from build123d import *

# Parameters (mm, degrees)
SKETCH1_W           = 133
SKETCH1_H           = 110
BOSS_EXTRUDE1_DEPTH = 3
SKETCH2_W           = 50
SKETCH2_H           = 18
SKETCH2_W_2         = 41
SKETCH2_H_2         = 15
SKETCH2_W_3         = 31
BOSS_EXTRUDE2_DEPTH = 3
CUT_EXTRUDE1_REACH  = 8
SKETCH3_R           = 15.25
SKETCH4_R           = 16.375
CUT_EXTRUDE2_DEPTH  = 1
CUT_EXTRUDE3_DEPTH  = 7
SKETCH7_W           = 15.45
SKETCH7_H           = 16.15
CUT_EXTRUDE4_DEPTH  = 1.5


with BuildPart() as part:
    # Sketch1 → Boss-Extrude1 (new body)
    with BuildSketch(Plane(origin=(0, 0, 0), x_dir=(1, 0, 0), z_dir=(0, 1, 0))):
        with Locations((66.5, 55)):
            Rectangle(SKETCH1_W, SKETCH1_H)
    extrude(amount=BOSS_EXTRUDE1_DEPTH)

    # Sketch2 → Boss-Extrude2 (add)
    with BuildSketch(Plane.XZ):
        with Locations((25, -109)):
            Rectangle(SKETCH2_W, SKETCH2_H)
        with Locations((112.5, -2.5)):
            Rectangle(SKETCH2_W_2, SKETCH2_H_2)
        with Locations((23.5, -2.5)):
            Rectangle(SKETCH2_W_3, SKETCH2_H_2)
    extrude(amount=BOSS_EXTRUDE2_DEPTH)

    # Sketch3 → Cut-Extrude1 (cut, up to next)
    with BuildSketch(Plane(origin=(0, 3, 0), x_dir=(1, 0, 0), z_dir=(0, 1, 0)), mode=Mode.PRIVATE) as cut_extrude1_sk1:
        with Locations((128.5, 28.75)):
            Circle(SKETCH3_R)
    cut_extrude1_tool1 = extrude(cut_extrude1_sk1.sketch, amount=-CUT_EXTRUDE1_REACH, mode=Mode.PRIVATE) & part.part
    add(cut_extrude1_tool1.solids().sort_by_distance((128.5, 3, -28.75))[0], mode=Mode.SUBTRACT)
    # Sketch3 → Cut-Extrude1 (cut, up to next)
    with BuildSketch(Plane(origin=(0, 3, 0), x_dir=(1, 0, 0), z_dir=(0, 1, 0)), mode=Mode.PRIVATE) as cut_extrude1_sk2:
        with Locations((135.5, 67.25)):
            Circle(SKETCH3_R)
    cut_extrude1_tool2 = extrude(cut_extrude1_sk2.sketch, amount=-CUT_EXTRUDE1_REACH, mode=Mode.PRIVATE) & part.part
    add(cut_extrude1_tool2.solids().sort_by_distance((135.5, 3, -67.25))[0], mode=Mode.SUBTRACT)

    # Sketch4 → Cut-Extrude2 (cut)
    with BuildSketch(Plane.XZ):
        with Locations((128.5, -28.75)):
            Circle(SKETCH4_R)
        with Locations((135.5, -67.25)):
            Circle(SKETCH4_R)
    extrude(amount=-CUT_EXTRUDE2_DEPTH, mode=Mode.SUBTRACT)

    # Sketch6 → Cut-Extrude3 (cut, through all)
    with BuildSketch(Plane(origin=(0, 3, 0), x_dir=(1, 0, 0), z_dir=(0, 1, 0))):
        Polygon((29.575, 84.225), (29.575, 78.275), (28.775, 78.275), (28.775, 74.175), (44.225, 74.175), (44.225, 78.275), (43.425, 78.275), (43.425, 84.225), (44.225, 84.225), (44.225, 88.325), (28.775, 88.325), (28.775, 84.225), align=None)
        Polygon((49.575, 84.225), (49.575, 78.275), (48.775, 78.275), (48.775, 74.175), (64.225, 74.175), (64.225, 78.275), (63.425, 78.275), (63.425, 84.225), (64.225, 84.225), (64.225, 88.325), (48.775, 88.325), (48.775, 84.225), align=None)
        Polygon((69.575, 79.225), (69.575, 73.275), (68.775, 73.275), (68.775, 69.175), (84.225, 69.175), (84.225, 73.275), (83.425, 73.275), (83.425, 79.225), (84.225, 79.225), (84.225, 83.325), (68.775, 83.325), (68.775, 79.225), align=None)
        Polygon((89.575, 39.225), (89.575, 33.275), (88.775, 33.275), (88.775, 29.175), (104.225, 29.175), (104.225, 33.275), (103.425, 33.275), (103.425, 39.225), (104.225, 39.225), (104.225, 43.325), (88.775, 43.325), (88.775, 39.225), align=None)
    extrude(amount=-CUT_EXTRUDE3_DEPTH, mode=Mode.SUBTRACT)

    # Sketch7 → Cut-Extrude4 (cut)
    with BuildSketch(Plane.XZ):
        with Locations((76.5, -76.25)):
            Rectangle(SKETCH7_W, SKETCH7_H)
        with Locations((96.5, -36.25)):
            Rectangle(SKETCH7_W, SKETCH7_H)
        with Locations((56.5, -81.25)):
            Rectangle(SKETCH7_W, SKETCH7_H)
        with Locations((36.5, -81.25)):
            Rectangle(SKETCH7_W, SKETCH7_H)
    extrude(amount=-CUT_EXTRUDE4_DEPTH, mode=Mode.SUBTRACT)


solid = part.part
The listing builds one solid part. Answer for the finished solid, in the listing's coordinates (mm). A direction names the side the tool comes from. Give positions to 0.01 mm unless a question says otherwise; leave off trailing zeros. Write each loop counter-clockwise with the first axis right and the second up, starting at its lowest first coordinate (ties: lowest second). Pieces come first, ordered by that corner, then holes. Notation, with made-up numbers: (47.25, 26) - (97.25, 26) arc R27 cw to (97.25, 45) - close; hole circle Ø11 at (-9.5, -5). An arc over 180 degrees is marked (long way). One line per question, with ' | ' between items. Start each with the question number.
1. Determine the mould class of faces 6 (the face through (112, -1, -10)), 7 (the face through (8, -1, -3)), 8 (the face through (120.253, 2.014, -67.55)), 9 (the face through (39, -1, -3)) for opening direction X: +X half, -X half, draft (parallel to the pull), parting line (faces both ways), or undercut.
2. For faces 1 (the face through (119.13, 0.49, -66.93)), 2 (the face through (25, 0, -114)), 3 (the face through (104.225, 1, -36)), 4 (the face through (25, -1, -100)), 5 (the face through (66, 1, 0)), determine the directions among +Z, -Z, +X, -X, +Y, -Y from which every point of the face is accessible in a straight line to the end or side of a thin tool.
3. Straight lines are drawn through the part: line 1 (Z direction, x = 10.5, y = -1.2); line 2 (Z direction, x = 94, y = 0.95) (3 decimals); line 3 (Z direction, x = 128.5, y = 0.7) (3 decimals). For each, find the intervals that lie inside material, in ascending order.
4. Section D-D, the plane z = -92 is taken. Determine the outline of the cut face in (x, y), then the cut area to 3 significant figures.
5. Section C-C, the plane z = -31.5 is taken. Determine the outline of the cut face in (x, y) (3 decimals), then the cut area to 3 significant figures.
6. Given P1, Ø1.2, axis at x = 37.5, y = 2.5, coming from the +Z side; P2, Ø1.5, axis at y = 2, z = -76.5, coming from the +X side; P3, Ø6, axis at x = 107.5, z = -22, coming from the -Y side; P4, Ø1, axis at y = -1, z = -97, coming from the -X side, each flat-ended and moving along its own axis, determine where each tip first touches the part or whether it passes through.
7. Section A-A, the plane x = 37.5 is taken. Determine the outline of the cut face in (y, z) (3 decimals), then the cut area to 3 significant figures.
8. Section B-B, the plane x = 128.5 is taken. Determine the outline of the cut face in (y, z) (3 decimals), then the cut area to 3 significant figures.
Result:
1) face 6: draft | face 7: -X half | face 8: +X half | face 9: undercut
2) face 1: +X, -Y | face 2: -Z, +X, -X, +Y | face 3: -Y | face 4: +X, -X, -Y | face 5: +Z, +X, -X, +Y
3) line 1: z = -118 to -100, -10 to 5 | line 2: z = -110 to -44.325, -28.175 to 0 | line 3: z = -110 to -82.053, -52.447 to -45.125, -12.375 to 0
4) outline: (0, 0) - (133, 0) - (133, 3) - (0, 3) - close | area: 399 mm2
5) outline: (0, 0) - (88.775, 0) - (88.775, 3) - (0, 3) - close; (104.225, 0) - (112.358, 0) - (112.358, 1) - (113.5, 1) - (113.5, 3) - (104.225, 3) - close | area: 293 mm2
6) P1: stops at z = 0 | P2: stops at x = 123.99 | P3: stops at y = 0 | P4: passes through
7) outline: (-3, -118) - (0, -118) - (0, -110) - (3, -110) - (3, -88.325) - (1.5, -88.325) - (1.5, -89.325) - (0, -89.325) - (0, -100) - (-3, -100) - close; (-3, -10) - (0, -10) - (0, -73.175) - (1.5, -73.175) - (1.5, -74.175) - (3, -74.175) - (3, 0) - (0, 0) - (0, 5) - (-3, 5) - close | area: 384 mm2
8) outline: (-3, -10) - (0, -10) - (0, -12.375) - (1, -12.375) - (1, -13.5) - (3, -13.5) - (3, 0) - (0, 0) - (0, 5) - (-3, 5) - close; (0, -110) - (3, -110) - (3, -80.799) - (1, -80.799) - (1, -82.053) - (0, -82.053) - close; (0, -52.447) - (1, -52.447) - (1, -53.701) - (3, -53.701) - (3, -44) - (1, -44) - (1, -45.125) - (0, -45.125) - close | area: 197 mm2
